```python
from build123d import *

# Parameters (mm, degrees)
SKETCH1_W           = 350
SKETCH1_H           = 100
SKETCH1_R           = 6
BOSS_EXTRUDE1_DEPTH = 3
SKETCH2_W           = 350
SKETCH2_H           = 40
BOSS_EXTRUDE2_DEPTH = 3
SKETCH3_R           = 4.15
CUT_EXTRUDE1_DEPTH  = 205.924376295
SKETCH4_R           = 1.25
CUT_EXTRUDE2_DEPTH  = 186.151289491


with BuildPart() as part:
    # Sketch1 → Boss-Extrude1 (new, symmetric)
    with BuildSketch(Plane(origin=(0, 0, 0), x_dir=(1, 0, 0), z_dir=(0, 1, 0))):
        Rectangle(SKETCH1_W, SKETCH1_H)
        with Locations(Location((143.57, 27.01502743, 0), (0, 0, 270))):
            Circle(SKETCH1_R, mode=Mode.SUBTRACT)
        with Locations(Location((-143.57, 27.01502743, 0), (0, 0, 270))):
            Circle(SKETCH1_R, mode=Mode.SUBTRACT)
    extrude(amount=BOSS_EXTRUDE1_DEPTH, both=True)

    # Sketch2 → Boss-Extrude2 (add)
    with BuildSketch(Plane.XY.offset(50)):
        with Locations((0, 17)):
            Rectangle(SKETCH2_W, SKETCH2_H)
    extrude(amount=-BOSS_EXTRUDE2_DEPTH)

    # Sketch3 → Cut-Extrude1 (cut, through all)
    with BuildSketch(Plane.XY.offset(50)):
        with Locations((0, 21.369646437)):
            Circle(SKETCH3_R)
    extrude(amount=-CUT_EXTRUDE1_DEPTH, mode=Mode.SUBTRACT)

    # Sketch4 → Cut-Extrude2 (cut, through all)
    with BuildSketch(Plane(origin=(0, 3, 0), x_dir=(1, 0, 0), z_dir=(0, 1, 0))):
        with Locations(Location((143.57, 37.01502743, 0), (0, 0, 270))):
            Circle(SKETCH4_R)
        with Locations(Location((153.57, 27.01502743, 0), (0, 0, 270))):
            Circle(SKETCH4_R)
        with Locations(Location((143.57, 17.01502743, 0), (0, 0, 270))):
            Circle(SKETCH4_R)
        with Locations(Location((133.57, 27.01502743, 0), (0, 0, 270))):
            Circle(SKETCH4_R)
        with Locations(Location((136.498932188, 34.086095242, 0), (0, 0, 270))):
            Circle(SKETCH4_R)
        with Locations(Location((150.641067812, 34.086095242, 0), (0, 0, 90))):
            Circle(SKETCH4_R)
        with Locations(Location((150.641067812, 19.943959618, 0), (0, 0, 270))):
            Circle(SKETCH4_R)
        with Locations(Location((136.498932188, 19.943959618, 0), (0, 0, 90))):
            Circle(SKETCH4_R)
    cut_extrude2 = extrude(amount=-CUT_EXTRUDE2_DEPTH, mode=Mode.SUBTRACT)

    # Mirror1: Cut-Extrude2 across plane
    add(cut_extrude2.mirror(Plane(origin=(0, 0, 0), x_dir=(0, 0, 1), z_dir=(1, 0, 0))), mode=Mode.SUBTRACT)


solid = part.part
```
Part model, mm, in its own coordinate system. A direction names the side the tool comes from. Round coordinates to 2 decimals unless told otherwise and drop trailing zeros. Loops run counter-clockwise (first coordinate to the right, second up) from the corner with the lowest first, then second, coordinate; pieces in that order, holes last. Notation, with made-up numbers: (44.25, 81.5) -> (67.25, 81.5) arc R20 cw to (67.25, 117.5) -> close; hole circle Ø4 at (49, -33.5). An arc over 180 degrees is marked (long way). Use CSV: the item, a comma, the result in double quotes. Start each with the question number.
1) Cut at D-D, the plane y = 12. Write the cut outline in (x, z), plus the area to 3 significant figures.
2) Cut at A-A, the plane x = 0. Write the cut outline in (y, z), plus the area to 3 significant figures.
3) Which spindle directions (+Z, -Z, +X, -X, +Y, -Y) get a long thin tool onto all of the face, cutting with end or side? Do faces 1 (the flat face through (175, 2, 8)), 2 (the flat face through (-2, 3, -2)). Say none if no direction does.
4) Cut at C-C, the plane z = 42.5. Write the cut outline in (x, y), plus the area to 3 significant figures.
5) Drop flat-ended pins along their axis: P1, Ø4, axis at x = 136.5, z = -34.09, coming from the +Y side; P2, Ø10, axis at x = 71.5, y = 19, coming from the -Z side. Give the stop position or say it passes through.
6) Pull direction Z, two halves, no side cores. Call faces 3 (the cylindrical face through (149.52, -0.04, -27.8)), 4 (the flat face through (-2, 0, -50)), 5 (the flat face through (-2, 17, 50)): +Z half, -Z half, draft (parallel to the pull), parting line (faces both ways), or undercut.
7) Wall check: L1, parallel to Z at x = 153.5, y = 0.5; L2, parallel to Y at x = -102, z = 25.5; L3, parallel to Z at x = 42, y = 19. Give the ranges that are in metal, low to high. Write a range as [from, to].
8) Cut at B-B, the plane x = 95. Write the cut outline in (y, z), plus the area to 3 significant figures.
Determined:
1,outline,"(-175, 47) -> (175, 47) -> (175, 50) -> (-175, 50) -> close"
1,area,"1,050 mm2"
2,outline,"(-3, -50) -> (3, -50) -> (3, 47) -> (17.22, 47) -> (17.22, 50) -> (-3, 50) -> close; (25.52, 47) -> (37, 47) -> (37, 50) -> (25.52, 50) -> close"
2,area,"677 mm2"
3,face 1,"+Z, -Z, +X, +Y, -Y"
3,face 2,"-Z, +X, -X, +Y"
4,outline,"(-175, -3) -> (175, -3) -> (175, 3) -> (-175, 3) -> close"
4,area,"2,100 mm2"
5,P1,"stops at y = 3"
5,P2,"stops at z = 47"
6,face 3,"undercut"
6,face 4,"-Z half"
6,face 5,"+Z half"
7,L1,"z = [-50, -28.26], [-25.77, 50]"
7,L2,"y = [-3, 3]"
7,L3,"z = [47, 50]"
8,outline,"(-3, -50) -> (3, -50) -> (3, 47) -> (37, 47) -> (37, 50) -> (-3, 50) -> close"
8,area,"702 mm2"
